Here's how the part is built. I have some questions about the finished solid (model axes, mm). Round coordinates to 2 decimals unless told otherwise and drop trailing zeros. Write each loop counter-clockwise with the first axis right and the second up, starting at its lowest first coordinate (ties: lowest second). Pieces come first, ordered by that corner, then holes. Notation, with made-up numbers: (59, 28.25) - (116, 28.25) arc R24 cw to (116, 58.25) - close; hole circle Ø5 at (42, 46.5). An arc over 180 degrees is marked (long way). One line per question, with ' | ' between items. Start each with the question number.
(1) Thinking about a two-plate mould opening in Z: for faces 1 (the cylindrical face through (6.571, -0.373, -81.137)), 2 (the cylindrical face through (11.976, -0.373, -0.764)), 3 (the cylindrical face through (6.78, -0.373, -114.623)), 4 (the flat face through (6, -0.737, -62)), which applies, pulls with the +Z half, pulls with the -Z half, needs draft (parallel to the pull), parting line crosses it, or undercut?
(2) Imagine slicing it at C-C (y = -0.6). Write out the boundary of the cut face in (x, z).
(3) Imagine slicing it at A-A (x = 6.35). Write out the boundary of the cut face in (y, z), plus the area to 3 significant figures.
(4) Imagine slicing it at B-B (z = -6.35). Write out the boundary of the cut face in (x, y).
(5) If I drill on L1, parallel to Z at x = 6.35, y = -0.3; L2, parallel to Z at x = 6, y = -0.6; L3, parallel to Z at x = 10.5, y = -0.3, over which ranges is the centre line in solid material (lowest first)?
(6) Will these pins go through, and if not, where does the flat tip stop? pin 1 (3 mm diameter, centred on x = 6.35, z = -116.56, fed in from -Y); pin 2 (4.5 mm diameter, centred on x = 6.35, z = -6.35, fed in from -Y).
from build123d import *

# Parameters (mm, degrees)
SKETCH1_W                       = 12.7
SKETCH1_H                       = 122.9106
BASE_FLANGE2_DEPTH              = 0.7366
M3_CLEARANCE_HOLE1_D            = 3.4
F_5_32_0_15625_DIAMETER_HOLE1_D = 3.96875
BREAK_CORNER1_START             = -0.7366
BREAK_CORNER1_DEPTH             = 0.7366


# Read off the part's stored shape, not the designer's step: Break-Corner1
# Sheet-metal steps are written as plain solids
with BuildPart() as part:
    # Sketch1 → Base-Flange2 (new body)
    with BuildSketch(Plane(origin=(0, 0, 0), x_dir=(1, 0, 0), z_dir=(0, 1, 0))):
        with Locations((6.35, 61.4553)):
            Rectangle(SKETCH1_W, SKETCH1_H)
    extrude(amount=-BASE_FLANGE2_DEPTH)

    # M3 Clearance Hole1 (through all)
    with Locations(Plane(origin=(0, 0, 0), x_dir=(1, 0, 0), z_dir=(0, 1, 0))):
        with Locations((6.35, 46.4512), (6.35, 79.4512)):
            Hole(M3_CLEARANCE_HOLE1_D / 2)

    # 5/32 (0.15625) Diameter Hole1 (through all)
    with Locations(Plane(origin=(0, 0, 0), x_dir=(1, 0, 0), z_dir=(0, 1, 0))):
        with Locations((6.35, 116.5606), (6.35, 6.35)):
            Hole(F_5_32_0_15625_DIAMETER_HOLE1_D / 2)

    # Break-Corner1 outline → Break-Corner1 (cut)
    with BuildSketch(Plane(origin=(0, 0, 0), x_dir=(1, 0, 0), z_dir=(0, 1, 0)).offset(BREAK_CORNER1_START)):
        with BuildLine():
            ThreePointArc((2.54, 0), (0.743948776, 0.743948776), (0, 2.54))
            Line((0, 2.54), (0, 0))
            Line((0, 0), (2.54, 0))
        make_face()
        with BuildLine():
            Line((0, 122.9106), (0, 120.3706))
            ThreePointArc((0, 120.3706), (0.743948776, 122.166651224), (2.54, 122.9106))
            Line((2.54, 122.9106), (0, 122.9106))
        make_face()
        with BuildLine():
            ThreePointArc((12.7, 2.54), (11.956051224, 0.743948776), (10.16, 0))
            Line((10.16, 0), (12.7, 0))
            Line((12.7, 0), (12.7, 2.54))
        make_face()
        with BuildLine():
            Line((12.7, 122.9106), (10.16, 122.9106))
            ThreePointArc((10.16, 122.9106), (11.956051224, 122.166651224), (12.7, 120.3706))
            Line((12.7, 120.3706), (12.7, 122.9106))
        make_face()
    extrude(amount=BREAK_CORNER1_DEPTH, mode=Mode.SUBTRACT)


solid = part.part
Check sheet entries:
1) face 1: undercut | face 2: pulls with the +Z half | face 3: undercut | face 4: needs draft
2) outline: (0, -120.37) arc R2.54 ccw to (2.54, -122.91) - (10.16, -122.91) arc R2.54 ccw to (12.7, -120.37) - (12.7, -2.54) arc R2.54 ccw to (10.16, 0) - (2.54, 0) arc R2.54 ccw to (0, -2.54) - close; hole circle Ø3.97 at (6.35, -116.56); hole circle Ø3.97 at (6.35, -6.35); hole circle Ø3.4 at (6.35, -79.45); hole circle Ø3.4 at (6.35, -46.45)
3) outline: (-0.74, -122.91) - (0, -122.91) - (0, -118.54) - (-0.74, -118.54) - close; (-0.74, -114.58) - (0, -114.58) - (0, -81.15) - (-0.74, -81.15) - close; (-0.74, -77.75) - (0, -77.75) - (0, -48.15) - (-0.74, -48.15) - close; (-0.74, -44.75) - (0, -44.75) - (0, -8.33) - (-0.74, -8.33) - close; (-0.74, -4.37) - (0, -4.37) - (0, 0) - (-0.74, 0) - close | area: 79.7 mm^2
4) outline: (0, -0.74) - (4.37, -0.74) - (4.37, 0) - (0, 0) - close; (8.33, -0.74) - (12.7, -0.74) - (12.7, 0) - (8.33, 0) - close
5) L1: -122.91 to -118.54, -114.58 to -81.15, -77.75 to -48.15, -44.75 to -8.33, -4.37 to 0 | L2: -122.91 to -118.51, -114.61 to -81.11, -77.79 to -48.11, -44.79 to -8.3, -4.4 to 0 | L3: -122.89 to -0.02
6) pin 1: through | pin 2: y = -0.74
